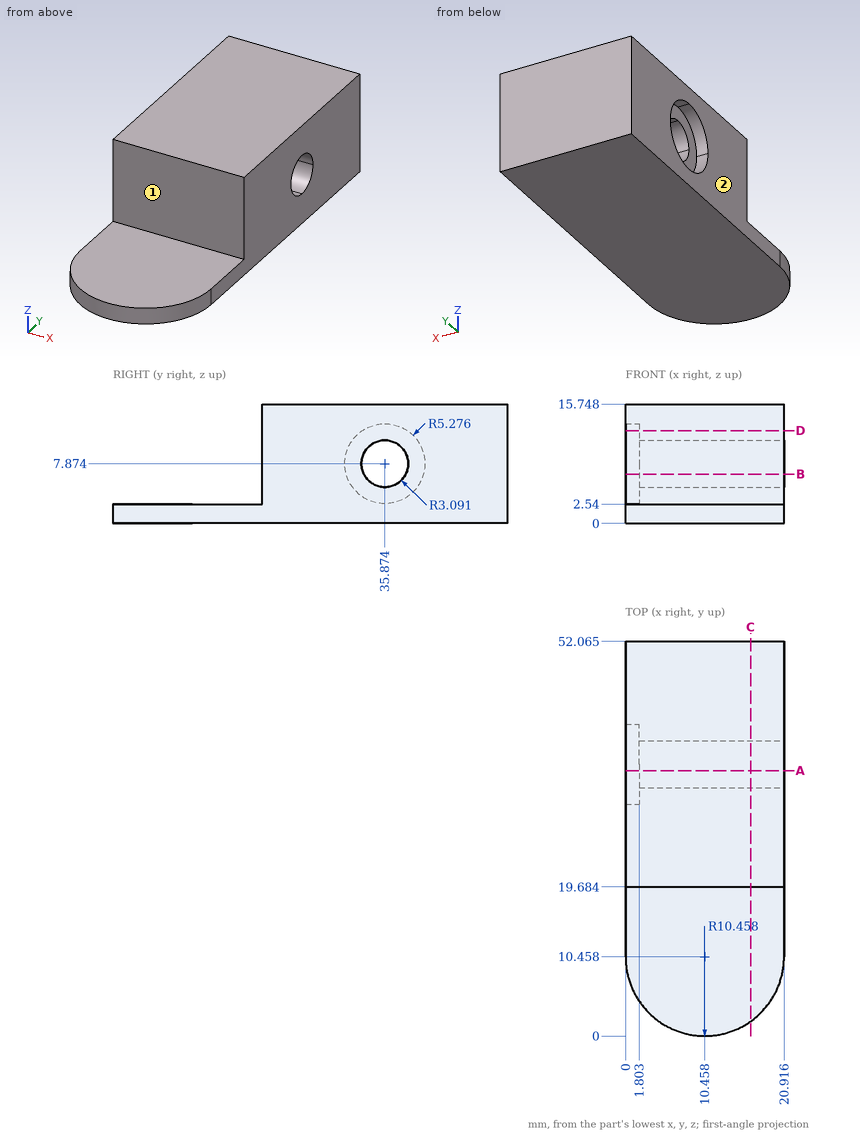
Input: dimensioned drawing with shaded views. Units: mm. Origin: part minimum x, y, z. A direction names the side the tool comes from. Coordinates: 2 decimals unless noted, no trailing zeros. Loops run counter-clockwise (first coordinate to the right, second up) from the corner with the lowest first, then second, coordinate; pieces in that order, holes last. Notation, with made-up numbers: (-8, 21) - (1, 21) arc R15 ccw to (1, 49) - close; hole circle Ø7 at (25, 31). An arc over 180 degrees is marked (long way). One line per question, with ' | ' between items. Start each with the question number.
(1) Cut plane D-D on z = 12.25. Output: boundary loops of the cut face in (x, y) (1 decimal).
(2) First-contact query: pin 1 (8 mm diameter, centred on x = 3.5, y = 21.5, fed in from -Z). Flat tip, straight axial feed; report the tip coordinate or a pass-through.
(3) Ray query, L1, parallel to Y at x = 2.25, z = 14.25 (1 decimal); L2, parallel to Z at x = 8.75, y = 10.5; L3, parallel to Y at x = 9, z = 9 (1 decimal). Return the intervals inside material, ascending. Write a range as from..to.
(4) Cut plane A-A on y = 35. Output: boundary loops of the cut face in (x, z), and give its area (3 significant figures).
(5) Cut plane C-C on x = 16.5. Output: boundary loops of the cut face in (y, z) (1 decimal).
(6) Cut plane B-B on z = 6.5. Output: boundary loops of the cut face in (x, y) (1 decimal), and give its area (3 significant figures).
(7) Reachability of the marked faces 1 and 2 from +Z, -Z, +X, -X, +Y, -Y: full face, straight path, thin tool, end or side. Return the list, or none.
Here are the results:
1) outline: (0, 19.7) - (20.9, 19.7) - (20.9, 52.1) - (0, 52.1) - (0, 38.8) - (1.8, 38.8) - (1.8, 32.9) - (0, 32.9) - close
2) pin 1: z = 0
3) L1: 19.7..52.1 | L2: 0..2.54 | L3: 19.7..33, 38.8..52.1
4) outline: (0, 0) - (20.92, 0) - (20.92, 4.91) - (1.8, 4.91) - (1.8, 2.67) - (0, 2.67) - close; (0, 13.08) - (1.8, 13.08) - (1.8, 10.84) - (20.92, 10.84) - (20.92, 15.75) - (0, 15.75) - close | area: 197 mm²
5) outline: (1.9, 0) - (52.1, 0) - (52.1, 15.7) - (19.7, 15.7) - (19.7, 2.5) - (1.9, 2.5) - close; hole circle Ø6.2 at (35.9, 7.9)
6) outline: (0, 19.7) - (20.9, 19.7) - (20.9, 33.1) - (1.8, 33.1) - (1.8, 30.8) - (0, 30.8) - close; (0, 41) - (1.8, 41) - (1.8, 38.6) - (20.9, 38.6) - (20.9, 52.1) - (0, 52.1) - close | area: 553 mm²
7) face 1: +Z, +X, -X, -Y | face 2: +Z, -Z, -X, +Y, -Y
